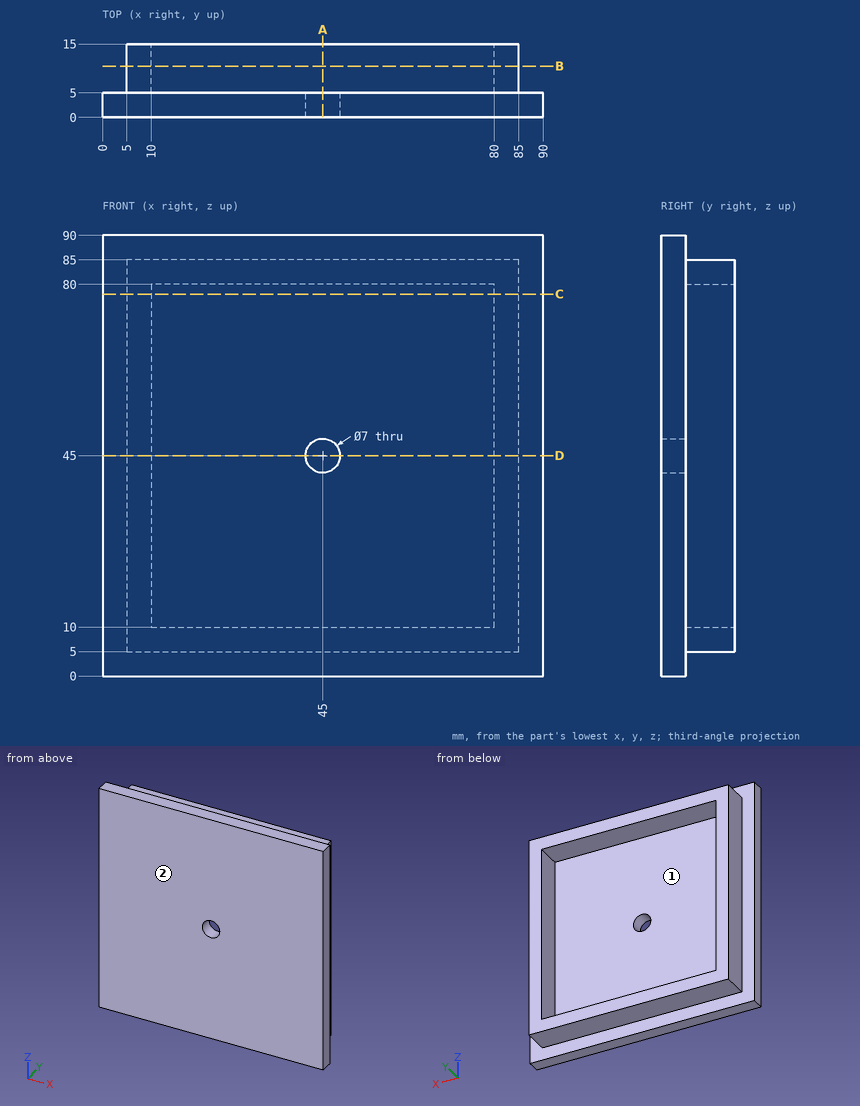
Could you check a few things on this drawing? It's one solid part, dimensions in mm from its lowest x, y, z. Give positions to 0.01 mm unless a question says otherwise; leave off trailing zeros. Order: outer loops, then holes, each group sorted by start corner. A loop starts at its lowest first (then second) coordinate and runs counter-clockwise, first axis right, second up. Notation, with made-up numbers: (-16, 79) -> (-11, 79) arc R20 cw to (-11, 87) -> close; hole circle Ø7 at (-15.75, 30). An arc over 180 degrees is marked (long way). Answer in a Markdown table with one row per item. Add a question column.
Item 1: Imagine slicing it at C-C (z = 78). List the corners of the cut face in (x, y) for me.
Item 2: Imagine slicing it at D-D (z = 45). List the corners of the cut face in (x, y) for me, and give its area (3 significant figures).
Item 3: We'd pull the mould along X, two halves only. Please class the marked faces 1 and 2: pulls with the +X half, pulls with the -X half, needs draft (parallel to the pull), parting line crosses it, or undercut.
Item 4: Imagine slicing it at B-B (y = 10.5). List the corners of the cut face in (x, z) for me.
Item 5: Imagine slicing it at A-A (x = 45). List the corners of the cut face in (y, z) for me, and give its area (3 significant figures).
Item 6: Please list where these lines run through material, in increasing order: probe 1 along X at (y, z) = (13.5, 71.5); probe 2 along Z at (x, y) = (45, 1.45).
Item 7: I'm going to push flat-ended pins straight in: P1, Ø3, axis at y = 10.5, z = 62, coming from the -X side; P2, Ø3, axis at x = 30.5, y = 9, coming from the -Z side; P3, Ø8, axis at y = 9.5, z = 42.5, coming from the +X side. Where does each tip first touch, or does it pass through?
Result:
| question | item | result |
|---|---|---|
| 1 | outline | (0, 0) -> (90, 0) -> (90, 5) -> (85, 5) -> (85, 15) -> (80, 15) -> (80, 5) -> (10, 5) -> (10, 15) -> (5, 15) -> (5, 5) -> (0, 5) -> close |
| 2 | outline | (0, 0) -> (41.5, 0) -> (41.5, 5) -> (10, 5) -> (10, 15) -> (5, 15) -> (5, 5) -> (0, 5) -> close; (48.5, 0) -> (90, 0) -> (90, 5) -> (85, 5) -> (85, 15) -> (80, 15) -> (80, 5) -> (48.5, 5) -> close |
| 2 | area | 515 mm2 |
| 3 | face 1 | undercut |
| 3 | face 2 | needs draft |
| 4 | outline | (5, 5) -> (85, 5) -> (85, 85) -> (5, 85) -> close; hole (10, 10) -> (80, 10) -> (80, 80) -> (10, 80) -> close |
| 5 | outline | (0, 0) -> (5, 0) -> (5, 5) -> (15, 5) -> (15, 10) -> (5, 10) -> (5, 41.5) -> (0, 41.5) -> close; (0, 48.5) -> (5, 48.5) -> (5, 80) -> (15, 80) -> (15, 85) -> (5, 85) -> (5, 90) -> (0, 90) -> close |
| 5 | area | 515 mm2 |
| 6 | probe 1 | 5 to 10, 80 to 85 |
| 6 | probe 2 | 0 to 41.5, 48.5 to 90 |
| 7 | P1 | x = 5 |
| 7 | P2 | z = 5 |
| 7 | P3 | x = 85 |
